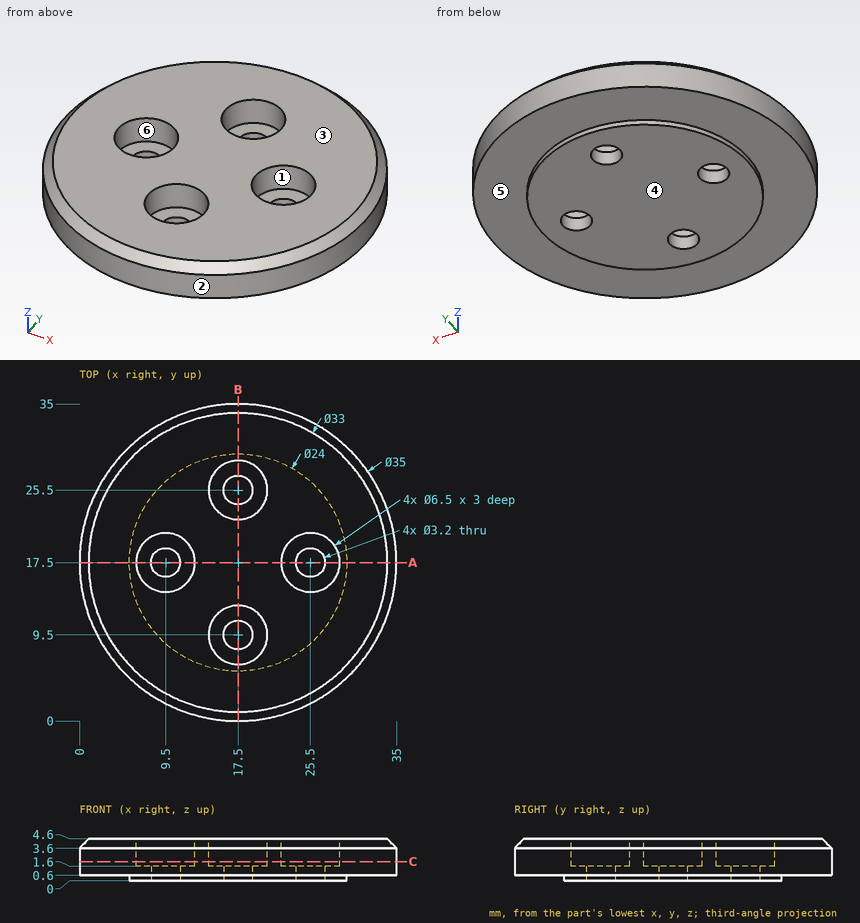
Answer from the drawing. Dimensions are ordinates in mm from the lowest x, y and z of the part. A direction names the side the tool comes from. Coordinates: 2 decimals unless noted, no trailing zeros. Loops run counter-clockwise (first coordinate to the right, second up) from the corner with the lowest first, then second, coordinate; pieces in that order, holes last. Notation, with made-up numbers: (59.5, 61) - (103.5, 61) arc R25 cw to (103.5, 96) - close; hole circle Ø6 at (79.5, 0.5). An arc over 180 degrees is marked (long way). Use a Markdown table: item, result.
Item 1: Find section C-C, the plane z = 2.1. Determine the outline of the cut face in (x, y).
Evaluation:
| item | result |
|---|---|
| outline | circle Ø35 at (17.5, 17.5); hole circle Ø6.5 at (9.5, 17.5); hole circle Ø6.5 at (17.5, 9.5); hole circle Ø6.5 at (17.5, 25.5); hole circle Ø6.5 at (25.5, 17.5) |
Item 2: Given pin 1 Ø7.5 at (x, y) = (9.5, 17.5) entering from -Z; pin 2 Ø4 at (x, y) = (25.5, 17.5) entering from +Z; pin 3 Ø1.9 at (x, y) = (17.5, 25.5) entering from +Z; pin 4 Ø1 at (x, y) = (29, 4) entering from -Z, each flat-ended and moving along its own axis, determine where each tip first touches the part or whether it passes through.
Evaluation:
| item | result |
|---|---|
| pin 1 | stops at z = 0 |
| pin 2 | stops at z = 1.6 |
| pin 3 | passes through |
| pin 4 | stops at z = 0.6 |
Item 3: For the marked faces 4, 5 and 6, determine the directions among +Z, -Z, +X, -X, +Y, -Y from which every point of the face is accessible in a straight line to the end or side of a thin tool.
Evaluation:
| item | result |
|---|---|
| face 4 | -Z, +X, -X, +Y, -Y |
| face 5 | -Z |
| face 6 | +Z |
Item 4: Consider probe 1 along Y at (x, z) = (17.5, 2.65); probe 2 along Y at (x, z) = (17.5, 0.55); probe 3 along X at (y, z) = (15.5, 4.45). Determine where each line is inside the solid, lowest interval first. Write a range as from..to.
Evaluation:
| item | result |
|---|---|
| probe 1 | y = 0..6.25, 12.75..22.25, 28.75..35 |
| probe 2 | y = 5.5..7.9, 11.1..23.9, 27.1..29.5 |
| probe 3 | x = 0.97..6.94, 12.06..22.94, 28.06..34.03 |
Item 5: The mould has two halves that part along Y. Classify the marked faces 1, 2 and 3: +Y half, -Y half, draft (parallel to the pull), parting line (faces both ways), or undercut.
Evaluation:
| item | result |
|---|---|
| face 1 | undercut |
| face 2 | parting line |
| face 3 | draft |
Item 6: Find section A-A, the plane y = 17.5. Determine the outline of the cut face in (x, z).
Evaluation:
| item | result |
|---|---|
| outline | (0, 0.6) - (5.5, 0.6) - (5.5, 0) - (7.9, 0) - (7.9, 1.6) - (6.25, 1.6) - (6.25, 4.6) - (1, 4.6) - (0, 3.6) - close; (11.1, 0) - (23.9, 0) - (23.9, 1.6) - (22.25, 1.6) - (22.25, 4.6) - (12.75, 4.6) - (12.75, 1.6) - (11.1, 1.6) - close; (27.1, 0) - (29.5, 0) - (29.5, 0.6) - (35, 0.6) - (35, 3.6) - (34, 4.6) - (28.75, 4.6) - (28.75, 1.6) - (27.1, 1.6) - close |
